from build123d import *

# Parameters (mm, degrees)
F0_R     = 15
F1_DEPTH = 30
F3_R     = 18
F4_DEPTH = 25
F5_R     = 15
F6_DEPTH = 3
F2_W     = 6
F2_H     = 6
F7_DEPTH = 35


with BuildPart() as f1:
    # F0 (on Top) → F1 (new body)
    with BuildSketch(Plane.XY):
        with BuildLine():
            ThreePointArc((-18.59375, -7.366985), (3.75, -19.645292), (20, 0))
            ThreePointArc((20, 0), (3.75, 19.645292), (-18.59375, 7.366985))
            ThreePointArc((-18.59375, 7.366985), (-20, 0), (-18.59375, -7.366985))
        make_face()
        Circle(F0_R, mode=Mode.SUBTRACT)
        with BuildLine():
            ThreePointArc((-18.59375, -7.366985), (-20, 0), (-18.59375, 7.366985))
            ThreePointArc((-18.59375, 7.366985), (-27.5, 0), (-18.59375, -7.366985))
        make_face()
        Circle(F0_R)
    extrude(amount=F1_DEPTH)

    # F3 (on face) → F4 (cut)
    with BuildSketch(Plane(origin=(0, 0, 0), x_dir=(1, 0, 0), z_dir=(0, 0, -1))):
        Circle(F3_R)
    extrude(amount=-F4_DEPTH, mode=Mode.SUBTRACT)

    # F5 (on face) → F6 (join)
    with BuildSketch(Plane.XY.offset(30)):
        Circle(F5_R)
    extrude(amount=F6_DEPTH)

    # F2 (on face) → F7 (cut)
    with BuildSketch(Plane.XY.offset(30)):
        with Locations((-22.077309, 0)):
            Rectangle(F2_W, F2_H)
    extrude(amount=-F7_DEPTH, mode=Mode.SUBTRACT)


solid = f1.part
Build history of the part. All positions in model axes, mm. A direction names the side the tool comes from. Coordinates: 2 decimals unless noted, no trailing zeros. Order: outer loops, then holes, each group sorted by start corner. A loop starts at its lowest first (then second) coordinate and runs counter-clockwise, first axis right, second up. Notation, with made-up numbers: (87.25, 12.25) - (145.25, 12.25) arc R11 ccw to (145.25, 19.25) - close; hole circle Ø1 at (56, -29.5). An arc over 180 degrees is marked (long way). Put each result on its own line as item: value.
1. Saw through at B-B (x = 0). Write the cut outline in (y, z).
Answer sheet:
outline: (-20, 0) - (-18, 0) - (-18, 25) - (18, 25) - (18, 0) - (20, 0) - (20, 30) - (15, 30) - (15, 33) - (-15, 33) - (-15, 30) - (-20, 30) - close
2. Drop flat-ended pins along their axis: P1, Ø5, axis at x = -22.5, z = 13.5, coming from the -Y side; P2, Ø5, axis at x = -4.5, z = 19.5, coming from the +Y side; P3, Ø1.5, axis at y = 12.5, z = 7.5, coming from the +X side. Give the stop position or say it passes through.
Answer sheet:
P1: stops at y = -7.5
P2: stops at y = 19.9
P3: stops at x = 16.18
3. Saw through at D-D (z = 21.5). Write the cut outline in (x, y), and give its area (3 significant figures).
Answer sheet:
outline: (-18.59, -7.37) arc R20 ccw (long way) to (-18.59, 7.37) arc R7.5 ccw (long way) to start; hole (-25.08, -3) - (-19.08, -3) - (-19.08, 3) - (-25.08, 3) - close; hole circle Ø36 at (0, 0)
area: 298 mm^2
4. Tool access for faces 1 (the face through (-13, 9, 30)), 2 (the face through (-18, -3, 0)), 3 (the face through (-2.343, -17.847, 12.325)), 4 (the face through (-22, -3, 15)): list every direction of +Z, -Z, +X, -X, +Y, -Y with a clear straight run to the whole face (end or side of a thin tool).
Answer sheet:
face 1: +Z
face 2: -Z, +X, -X, +Y, -Y
face 3: -Z
face 4: +Z, -Z
5. Saw through at C-C (z = 27.5). Write the cut outline in (x, y), and give its area (3 significant figures).
Answer sheet:
outline: (-18.59, -7.37) arc R20 ccw (long way) to (-18.59, 7.37) arc R7.5 ccw (long way) to start; hole (-25.08, -3) - (-19.08, -3) - (-19.08, 3) - (-25.08, 3) - close
area: 1,320 mm^2
6. Probe line 1 along X through (y, z) = (0, 14.25); line 2 along Z through (x, y) = (3, 6.5); line 3 along Z through (x, y) = (7.5, 14). List the from-to ranges inside material, lowest first. Write a range as [from, to].
Answer sheet:
line 1: x = [-27.5, -25.08], [-19.08, -18], [18, 20]
line 2: z = [25, 33]
line 3: z = [25, 30]
7. Pull direction X, two halves, no side cores. Call faces 5 (the face through (0, 0, 33)), 6 (the face through (-14.985, 0.66, 31.479)), 7 (the face through (-25.077, 0, 15)): pulls with the +X half, pulls with the -X half, needs draft (parallel to the pull), parting line crosses it, or undercut.
Answer sheet:
face 5: needs draft
face 6: parting line crosses it
face 7: undercut
8. Saw through at A-A (x = -20). Write the cut outline in (y, z).
Answer sheet:
outline: (-7.5, 0) - (-3, 0) - (-3, 30) - (-7.5, 30) - close; (3, 0) - (7.5, 0) - (7.5, 30) - (3, 30) - close
